The model under review builds one solid part; all positions refer to its coordinate system, in mm. A direction names the side the tool comes from. Coordinates: 2 decimals unless noted, no trailing zeros. Loops run counter-clockwise (first coordinate to the right, second up) from the corner with the lowest first, then second, coordinate; pieces in that order, holes last. Notation, with made-up numbers: (-36.75, -18.75) - (-13.75, -18.75) arc R29 cw to (-13.75, 1.25) - close; hole circle Ø11 at (10.5, 70). An arc over 180 degrees is marked (long way). One line per item, written item: value. Start each with the question number.
1. We need section A-A, the plane y = -3. Give the boundary of the cut face in (x, z) (1 decimal).
2. Mouldability with a two-part tool opening along Y and no side actions: class faces 1 (the face through (85.285, 2.861, 12.878)), 2 (the face through (14.288, 0, 65)), 3 (the face through (-27.17, 1.38, 50.95)), 4 (the face through (-1, 25.4, 32)) as +Y half, -Y half, draft (parallel to the pull), parting line (faces both ways), or undercut.
3. To check wall thickness, follow line 1 (X direction, y = 11, z = 50); line 2 (Z direction, x = -23.5, y = 0); line 3 (Z direction, x = 74, y = -32). State the ranges of each line that lie inside material, in increasing order.
4. Insertion check: P1, Ø20.5, axis at y = 0, z = 57.15, coming from the +X side; P2, Ø5, axis at y = 23, z = 33, coming from the -X side; P3, Ø5, axis at x = -32, z = 47, coming from the +Y side; P4, Ø10, axis at y = 0, z = 57.15, coming from the -X side. Each pin has a flat end and moves straight along its axis. Give the tip position at first contact, or say it passes through.
5. We need section B-B, the plane z = 14. Give the boundary of the cut face in (x, y) (3 decimals), then the cut area to 3 significant figures.
6. We need section D-D, the plane z = 57.15. Give the boundary of the cut face in (x, y).
7. For faces 5 (the face through (-1, -25.4, 32)), 6 (the face through (-14.288, 0, 65)), 7 (the face through (39.688, 0, 50)), list the 3-axis set-ups (+Z, -Z, +X, -X, +Y, -Y) from which the entire face can be reached by the end or side of a thin tool; tool diameter is ignored.
8. We need section C-C, the plane x = 0. Give the boundary of the cut face in (y, z).
from build123d import *

# Parameters (mm, degrees)
F1_DEPTH  = 25.4
F2_W      = 79.375
F2_H      = 50.8
F3_DEPTH  = 50.8
F5_DEPTH  = 63.501
F6_R      = 25.39999
F7_R      = 6.35
F8_DEPTH  = 127
F9_R      = 9.525
F10_DEPTH = 25.401


# Not quite as in the source:
# - a fillet or chamfer is up to 0.001 mm smaller than in the source, because OpenCascade refuses the exact size


with BuildPart() as f1:
    # F0 (on Top) → F1 (new body)
    with BuildSketch(Plane.XY):
        with BuildLine():
            ThreePointArc((76.2, -38.1), (114.3, 0), (76.2, 38.1))
            Line((76.2, 38.1), (-76.2, 38.1))
            ThreePointArc((-76.2, 38.1), (-114.3, 0), (-76.2, -38.1))
            Line((-76.2, -38.1), (76.2, -38.1))
        make_face()
    extrude(amount=F1_DEPTH)

    # F2 (on face) → F3 (join)
    with BuildSketch(Plane.XY.offset(25.4)):
        Rectangle(F2_W, F2_H)
    extrude(amount=F3_DEPTH)

    # F4 (on face) → F5 (cut, through all)
    with BuildSketch(Plane.XZ.offset(25.4)):
        with BuildLine():
            Line((14.2875, 76.2), (-14.2875, 76.2))
            Line((-14.2875, 76.2), (-14.2875, 47.625))
            ThreePointArc((-14.2875, 47.625), (0, 33.3375), (14.2875, 47.625))
            Line((14.2875, 47.625), (14.2875, 76.2))
        make_face()
    extrude(amount=-F5_DEPTH, mode=Mode.SUBTRACT)

    # F6 (radius 25.4 in the source; OpenCascade refuses exactly that, so slightly less here)
    f6_edges = [f1.edges().sort_by_distance(p)[0] for p in [
        (-26.9875, -25.4, 76.2),
        (-26.9875, 25.4, 76.2),
        (26.9875, -25.4, 76.2),
        (26.9875, 25.4, 76.2),
    ]]
    fillet(f6_edges, radius=F6_R)

    # F7 (on face) → F8 (cut)
    with BuildSketch(Plane(origin=(-39.6875, 0, 0), x_dir=(0, -1, 0), z_dir=(-1, 0, 0))):
        with Locations((0, 57.15)):
            Circle(F7_R)
    extrude(amount=-F8_DEPTH, mode=Mode.SUBTRACT)

    # F9 (on face) → F10 (cut, through all)
    with BuildSketch(Plane.XY.offset(25.4)):
        with Locations((-76.2, 0)):
            Circle(F9_R)
        with Locations((76.2, 0)):
            Circle(F9_R)
    extrude(amount=-F10_DEPTH, mode=Mode.SUBTRACT)


solid = f1.part
Findings below:
1. outline: (-114.2, 0) - (-85.2, 0) - (-85.2, 25.4) - (-114.2, 25.4) - close; (-67.2, 0) - (67.2, 0) - (67.2, 25.4) - (39.7, 25.4) - (39.7, 51.6) - (14.3, 51.6) - (14.3, 47.6) arc R14.3 cw to (-14.3, 47.6) - (-14.3, 51.6) - (-39.7, 51.6) - (-39.7, 25.4) - (-67.2, 25.4) - close; (-39.7, 62.7) - (-14.3, 62.7) - (-14.3, 76) - (-39.7, 76) - close; (14.3, 62.7) - (39.7, 62.7) - (39.7, 76) - (14.3, 76) - close; (85.2, 0) - (114.2, 0) - (114.2, 25.4) - (85.2, 25.4) - close
2. face 1: undercut
2. face 2: draft
2. face 3: undercut
2. face 4: +Y half
3. line 1: -39.69 to -14.29, 14.29 to 39.69
3. line 2: 0 to 50.8, 63.5 to 76.2
3. line 3: 0 to 25.4
4. P1: x = 39.69
4. P2: x = -39.69
4. P3: y = 25.4
4. P4: through
5. outline: (-76.2, -38.1) - (76.2, -38.1) arc R38.1 ccw to (76.2, 38.1) - (-76.2, 38.1) arc R38.1 ccw to start; hole circle Ø19.05 at (-76.2, 0); hole circle Ø19.05 at (76.2, 0)
5. area: 15,600 mm2
6. outline: (-39.69, -24.59) - (-14.29, -24.59) - (-14.29, -6.35) - (-39.69, -6.35) - close; (-39.69, 6.35) - (-14.29, 6.35) - (-14.29, 24.59) - (-39.69, 24.59) - close; (14.29, -24.59) - (39.69, -24.59) - (39.69, -6.35) - (14.29, -6.35) - close; (14.29, 6.35) - (39.69, 6.35) - (39.69, 24.59) - (14.29, 24.59) - close
7. face 5: +Z, +X, -X, -Y
7. face 6: +Z, +Y, -Y
7. face 7: +Z, +X, +Y, -Y
8. outline: (-38.1, 0) - (38.1, 0) - (38.1, 25.4) - (25.4, 25.4) - (25.4, 33.34) - (-25.4, 33.34) - (-25.4, 25.4) - (-38.1, 25.4) - close
